Can you work these out from the drawing? Everything is in mm from the part's minimum corner. A direction names the side the tool comes from. Round coordinates to 2 decimals unless told otherwise and drop trailing zeros. Write each loop counter-clockwise with the first axis right and the second up, starting at its lowest first coordinate (ties: lowest second). Pieces come first, ordered by that corner, then holes. Notation, with made-up numbers: (-25, 48) -> (-20, 48) arc R19 cw to (-20, 58) -> close; hole circle Ø7 at (82, 17.5). An arc over 180 degrees is marked (long way). Put each result on its own line as item: value. Start each with the question number.
1. Suppose I cut it at A-A (x = 14.25). Please give me the cut outline in (y, z), then the cut area to 3 significant figures.
2. For pin 1 (2.5 mm diameter, centred on x = 13, z = 6, fed in from -Y); pin 2 (2 mm diameter, centred on x = 16, y = 5, fed in from -Z); pin 3 (1 mm diameter, centred on y = 3, z = 5.5, fed in from -X); pin 4 (2 mm diameter, centred on x = 9.5, y = 2.5, fed in from +Z), each with a flat end and sliding along its axis, tell me the tip position at first contact or that it passes through.
3. Suppose I cut it at B-B (z = 1.25). Please give me the cut outline in (x, y), then the cut area to 3 significant figures.
4. We'd pull the mould along Z, two halves only. Please class the marked faces 1, 2 and 3: +Z half, -Z half, draft (parallel to the pull), parting line (faces both ways), or undercut.
5. I need wall thicknesses on probe 1 along Z at (x, y) = (9, 5.5); probe 2 along Y at (x, z) = (16, 1); probe 3 along Z at (x, y) = (8, 4.25). Which ranges of each line are inside material? Lowest first, please. Write a range as from..to.
6. Which directions (+Z, -Z, +X, -X, +Y, -Y) give clear straight access to the entire face, cutting with the end or side of a thin tool? Please do the marked faces 4, 5, 6 and 7.
7. Suppose I cut it at C-C (x = 7.25). Please give me the cut outline in (y, z), then the cut area to 3 significant figures.
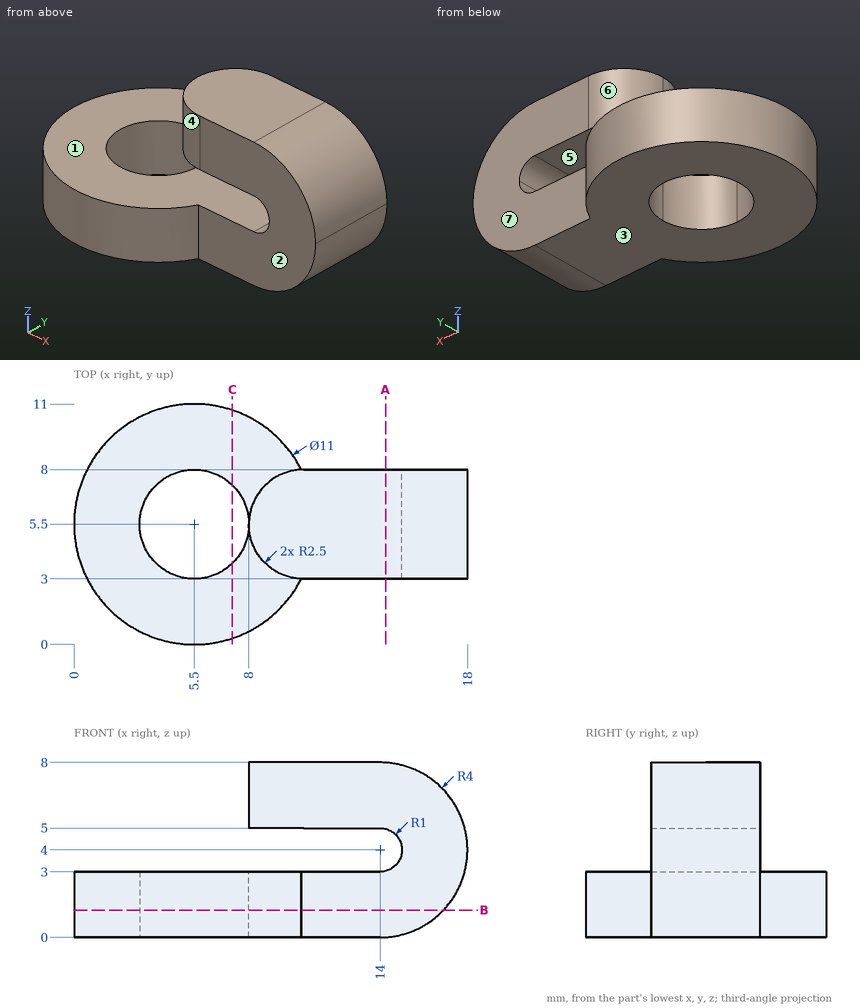
Verdict:
1. outline: (3, 0.01) -> (8, 0.01) -> (8, 3.03) -> (3, 3.03) -> close; (3, 4.97) -> (8, 4.97) -> (8, 7.99) -> (3, 7.99) -> close
1. area: 30.2 mm^2
2. pin 1: stops at y = 3
2. pin 2: stops at z = 0.13
2. pin 3: stops at x = 9
2. pin 4: stops at z = 8
3. outline: (10.4, 3) -> (16.9, 3) -> (16.9, 8) -> (10.4, 8) arc R5.5 ccw (long way) to start; hole circle Ø5 at (5.5, 5.5)
3. area: 106 mm^2
4. face 1: undercut
4. face 2: draft
4. face 3: -Z half
5. probe 1: z = 0..3, 5..8
5. probe 2: y = 3..8
5. probe 3: z = 0..3
6. face 4: +Z, -X, -Y
6. face 5: -X, +Y, -Y
6. face 6: +Z, -X, +Y
6. face 7: +Z, -Z, +X, +Y
7. outline: (0.29, 0) -> (3.71, 0) -> (3.71, 3) -> (0.29, 3) -> close; (7.29, 0) -> (10.71, 0) -> (10.71, 3) -> (7.29, 3) -> close
7. area: 20.6 mm^2
